from build123d import *

# Parameters (mm, degrees)
BOSS_EXTRUDE1_DEPTH = 10
FILLET1_R           = 25
SKETCH3_W           = 70
SKETCH3_H           = 80
BOSS_EXTRUDE2_DEPTH = 24.5


# Read off the part's stored shape, not the designer's step: Boss-Extrude1
with BuildPart() as part:
    # Boss-Extrude1 outline → Boss-Extrude1 (new body)
    with BuildSketch(Plane(origin=(0, 0, 0), x_dir=(1, 0, 0), z_dir=(0, 1, 0))):
        with BuildLine():
            Line((-250, -100), (-170, -100))
            add(Edge.make_bspline(
                [(-170, -100), (-120, -100), (-100, -130), (-70, -145), (-45, -145)],
                knots=[0, 0, 0, 0, 0, 1, 1, 1, 1, 1], degree=4))
            Line((-45, -145), (45, -145))
            add(Edge.make_bspline(
                [(45, -145), (70, -145), (100, -130), (120, -100), (170, -100)],
                knots=[0, 0, 0, 0, 0, 1, 1, 1, 1, 1], degree=4))
            Line((170, -100), (250, -100))
            Line((250, -100), (250, 100))
            Line((250, 100), (170, 100))
            add(Edge.make_bspline(
                [(170, 100), (120, 100), (100, 130), (70, 145), (45, 145)],
                knots=[0, 0, 0, 0, 0, 1, 1, 1, 1, 1], degree=4))
            Line((45, 145), (-45, 145))
            add(Edge.make_bspline(
                [(-45, 145), (-70, 145), (-100, 130), (-120, 100), (-170, 100)],
                knots=[0, 0, 0, 0, 0, 1, 1, 1, 1, 1], degree=4))
            Line((-170, 100), (-250, 100))
            Line((-250, 100), (-250, -100))
        make_face()
    extrude(amount=BOSS_EXTRUDE1_DEPTH)

    # Fillet1
    fillet1_edges = [part.edges().sort_by_distance(p)[0] for p in [
        (-250, 5, 100),
        (-250, 5, -100),
        (250, 5, -100),
        (250, 5, 100),
    ]]
    fillet(fillet1_edges, radius=FILLET1_R)

    # Sketch3 → Boss-Extrude2 (add)
    with BuildSketch(Plane.XZ):
        with Locations((0, -105)):
            Rectangle(SKETCH3_W, SKETCH3_H)
        with Locations((0, 105)):
            Rectangle(SKETCH3_W, SKETCH3_H)
    extrude(amount=BOSS_EXTRUDE2_DEPTH)


solid = part.part
CAD build for the part. Positions are in the model's coordinates, mm. A direction names the side the tool comes from. Round coordinates to 2 decimals unless told otherwise and drop trailing zeros. Order: outer loops, then holes, each group sorted by start corner. A loop starts at its lowest first (then second) coordinate and runs counter-clockwise, first axis right, second up. Notation, with made-up numbers: (9.25, 62.25) -> (39.25, 62.25) arc R34 ccw to (39.25, 92.25) -> close; hole circle Ø10 at (20, 75). An arc over 180 degrees is marked (long way). Write each question's results on one line, items separated by ' | '.
1. Wall check: line 1 along X through (y, z) = (-16.5, 76.5); line 2 along Y through (x, z) = (84.5, -17); line 3 along Z through (x, y) = (106, 6). Give the ranges that are in metal, low to high. Write a range as [from, to].
Findings below:
line 1: x = [-35, 35] | line 2: y = [0, 10] | line 3: z = [-120.77, 120.77]
2. Cut at A-A (y = -19). Give the cut face in (x, z).
Findings below:
outline: (-35, -145) -> (35, -145) -> (35, -65) -> (-35, -65) -> close; (-35, 65) -> (35, 65) -> (35, 145) -> (-35, 145) -> close
3. Cut at C-C (z = 86.5). Give the cut face in (x, y).
Findings below:
outline: (-247.2, 0) -> (-35, 0) -> (-35, -24.5) -> (35, -24.5) -> (35, 0) -> (247.2, 0) -> (247.2, 10) -> (-247.2, 10) -> close
4. Cut at B-B (x = -195). Give the cut face in (y, z).
Findings below:
outline: (0, -100) -> (10, -100) -> (10, 100) -> (0, 100) -> close
5. 3-axis set-ups, long thin cutter, end or side, ignore diameter. For faces 1 (the face through (-35, -12, 104)), 2 (the face through (242.482, 5.07, 92.871)), 3 (the face through (0, -24.5, -104)), 4 (the face through (35, -12, -106)), 5 (the face through (198, 5, -100)): which of +Z, -Z, +X, -X, +Y, -Y reach the whole face in a straight line?
Findings below:
face 1: +Z, -Z, -X, -Y | face 2: +Z, +X, +Y, -Y | face 3: +Z, -Z, +X, -X, -Y | face 4: +Z, -Z, +X, -Y | face 5: -Z, +X, +Y, -Y
6. Flat gauge pins, fed straight in: P1, Ø3, axis at x = -187, y = 5, coming from the +Z side; P2, Ø12, axis at y = 1, z = -102, coming from the +X side; P3, Ø19.5, axis at y = -14, z = -122.5, coming from the +X side. Where does each tip first touch, or does it go through?
Findings below:
P1: stops at z = 100 | P2: stops at x = 238.56 | P3: stops at x = 35
7. Cut at D-D (z = -39.5). Give the cut face in (x, y).
Findings below:
outline: (-250, 0) -> (250, 0) -> (250, 10) -> (-250, 10) -> close
8. Pull direction Z, two halves, no side cores. Call faces 6 (the face through (0, -12, 65)), 7 (the face through (197, 5, 100)), 8 (the face through (-3, 10, -2)): pulls with the +Z half, pulls with the -Z half, needs draft (parallel to the pull), parting line crosses it, or undercut.
Findings below:
face 6: undercut | face 7: pulls with the +Z half | face 8: needs draft
